Geometry: final body of the model. Coordinates: model frame, mm. Give positions to 0.01 mm unless a question says otherwise; leave off trailing zeros. Write each loop counter-clockwise with the first axis right and the second up, starting at its lowest first coordinate (ties: lowest second). Pieces come first, ordered by that corner, then holes.
Q1. Section B-B (z = 2.5). Return the cut outline in (x, y).
Q2. Section C-C (x = -16.5). Return the cut outline in (y, z).
Q3. Section D-D (z = 8.5). Return the cut outline in (x, y).
Q4. Section A-A (x = -48.75). Return the cut outline in (y, z).
Q5. Pin query (flat end, axial travel): pin 1 Ø1.8 at (x, z) = (20.25, -8.5) entering from +Y. Return the tip coordinate at first contact, or that it passes through.
Q6. Line query: line 1 (Z direction, x = -48.75, y = 0.75); line 2 (X direction, y = 1, z = 8.5); line 3 (Z direction, x = 9, y = 3.25). Output: solid intervals per line, ascending.
Autodesk Inventor part; units mm, degrees
ref_plane "YZ Plane" through (0, 0, 0) normal (1, 0, 0) x (0, 1, 0)
ref_plane "XZ Plane" through (0, 0, 0) normal (0, 1, 0) x (-1, 0, 0)
ref_plane "XY Plane" through (0, 0, 0) normal (0, 0, 1) x (1, 0, 0)
sketch "Sketch1" plane through (0, 0, 0) normal (0, 1, 0) x (-1, 0, 0)
  line L0 (0, 0) -> (-16.25, 0)
  line L1 (0, 0) -> (44.75, 0)
  line L2 (300, 0) -> (330, 0) construction
  line L3 (330, 30) -> (-30, 30) construction
  line L4 (-16.25, 15.5) -> (44.75, 15.5)
  line L5 (44.75, 15.5) -> (44.75, 0)
  line L6 (44.75, -15.5) -> (-16.25, -15.5)
  line L7 (-16.25, -15.5) -> (-16.25, 0)
  line L8 (-16.25, 15.5) -> (44.75, -15.5) construction
  line L9 (44.75, 15.5) -> (-16.25, -15.5) construction
  line L10 (-20.25, 8.5) -> (48.75, 8.5) construction
  line L11 (48.75, 8.5) -> (48.75, -8.5) construction
  line L12 (48.75, -8.5) -> (-20.25, -8.5) construction
  line L13 (-20.25, -8.5) -> (-20.25, 8.5) construction
  line L14 (-20.25, 8.5) -> (48.75, -8.5) construction
  line L15 (48.75, 8.5) -> (-20.25, -8.5) construction
  line L16 (-30, 0) -> (-30, 30)
  line L17 (330, 0) -> (330, 30) construction
  line L18 (44.75, 0) -> (300, 0) construction
  line L19 (44.75, 0) -> (44.75, -15.5)
  line L20 (-16.25, 0) -> (-30, 0)
  line L21 (-16.25, 0) -> (-16.25, 15.5)
  line L22 (300, 0) -> (300, 18.5) construction
  line L23 (0, 0) -> (-30, 0) construction
  line L24 (44.75, 0) -> (59.75, 0)
  line L25 (59.75, 0) -> (59.75, 30)
  line L26 (-30, 30) -> (59.75, 30)
  point P0 (14.25, 0)
  point P1 (14.25, 0)
  point P2 (285, 0)
  dimension "d0" = 300
  dimension "d5" = 61
  dimension "d6" = 31
  dimension "d7" = 69
  dimension "d8" = 17
  dimension "d9" = 16.25
  dimension "d10" = 30
  dimension "d11" = 30
  dimension "d20" = 18.5
  dimension "d21" = 15
  dimension "d29" = 15
extrude "Extrusion1" add sketch "Sketch1" along normal blind 3.5 contours L20 L16 L26 L25 L24 L5 L4 L21
hole "Hole1" at (20.25, 0, 8.5) at (-48.75, 0, 8.5) direction (0, 1, 0) diameter 2 end through all
fillet "Fillet1" radius 20 1 edges at (30, 1.75, 30)
mirror "Mirror1" about plane through (30, 0, 0) normal (0, 0, -1)
properties part number "segment1c" material "Plywood, Finish"
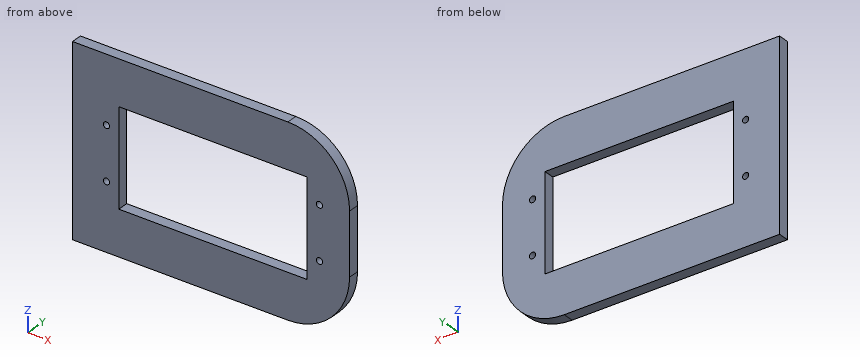
Computed:
1. outline: (-59.75, 0) - (-44.75, 0) - (-44.75, 3.5) - (-59.75, 3.5) - close; (16.25, 0) - (30, 0) - (30, 3.5) - (16.25, 3.5) - close
2. outline: (0, -30) - (3.5, -30) - (3.5, -15.5) - (0, -15.5) - close; (0, 15.5) - (3.5, 15.5) - (3.5, 30) - (0, 30) - close
3. outline: (-59.75, 0) - (-49.75, 0) - (-49.75, 3.5) - (-59.75, 3.5) - close; (-47.75, 0) - (-44.75, 0) - (-44.75, 3.5) - (-47.75, 3.5) - close; (16.25, 0) - (19.25, 0) - (19.25, 3.5) - (16.25, 3.5) - close; (21.25, 0) - (30, 0) - (30, 3.5) - (21.25, 3.5) - close
4. outline: (0, -30) - (3.5, -30) - (3.5, -9.5) - (0, -9.5) - close; (0, -7.5) - (3.5, -7.5) - (3.5, 7.5) - (0, 7.5) - close; (0, 9.5) - (3.5, 9.5) - (3.5, 30) - (0, 30) - close
5. pin 1: passes through
6. line 1: z = -30 to -9.5, -7.5 to 7.5, 9.5 to 30
6. line 2: x = -59.75 to -49.75, -47.75 to -44.75, 16.25 to 19.25, 21.25 to 30
6. line 3: z = -30 to -15.5, 15.5 to 30
